Autodesk Inventor part; units mm, degrees
ref_plane "YZ Plane" through (0, 0, 0) normal (1, 0, 0) x (0, 1, 0)
ref_plane "XZ Plane" through (0, 0, 0) normal (0, 1, 0) x (-1, 0, 0)
ref_plane "XY Plane" through (0, 0, 0) normal (0, 0, 1) x (1, 0, 0)
sketch "Sketch1" plane through (0, 0, 0) normal (0, 1, 0) x (-1, 0, 0)
  line L0 (-21.15, 21.15) -> (21.15, 21.15)
  line L1 (21.15, 21.15) -> (21.15, -21.15)
  line L2 (21.15, -21.15) -> (-21.15, -21.15)
  line L3 (-21.15, -21.15) -> (-21.15, 21.15)
  line L4 (-21.15, 21.15) -> (21.15, -21.15) construction
  line L5 (21.15, 21.15) -> (-21.15, -21.15) construction
  line L6 (-15.5, 15.5) -> (15.5, 15.5)
  line L7 (15.5, 15.5) -> (15.5, -15.5)
  line L8 (15.5, -15.5) -> (-15.5, -15.5)
  line L9 (-15.5, -15.5) -> (-15.5, 15.5)
  line L10 (-15.5, 15.5) -> (15.5, -15.5) construction
  line L11 (15.5, 15.5) -> (-15.5, -15.5) construction
  line L12 (15.5, -21.15) -> (21.15, -15.5)
  line L13 (-21.15, -15.5) -> (-15.5, -21.15)
  line L14 (-21.15, 15.5) -> (-15.5, 21.15)
  line L15 (15.5, 21.15) -> (21.15, 15.5)
  point P0 (0, 0)
  dimension "d0" = 42.3
  dimension "d1" = 42.3
  dimension "d2" = 31
  dimension "d3" = 31
  dimension "d4" = 31
  dimension "d5" = 31
  dimension "d6" = 31
  dimension "d7" = 31
  dimension "d8" = 45
extrude "Extrusion1" add sketch "Sketch1" along normal blind 48 contours L0 L15 L1 L12 L2 L13 L3 L14 | L6 L7 L8 L9
sketch "Sketch2" plane through (0, 48, 0) normal (0, 1, 0) x (1, 0, 0)
  circle A0 centre (0, 0) radius 11
  dimension "d11" = 22
extrude "Extrusion2" add sketch "Sketch2" along normal blind 2
sketch "Sketch3" plane through (0, 50, 0) normal (0, 1, 0) x (1, 0, 0)
  circle A0 centre (0, 0) radius 2.5
  dimension "d14" = 5
extrude "Extrusion3" add sketch "Sketch3" along normal blind 22
sketch "Sketch4" plane through (0, 72, 0) normal (0, 1, 0) x (1, 0, 0)
  circle A0 centre (0, 0) radius 2.5
  line L0 (-1.5, 2) -> (1.5, 2)
  circle A1 centre (0, 0) radius 2.5
  dimension "d21" = 5
  dimension "d20" = 2
extrude "Extrusion4" cut sketch "Sketch4" against normal blind 15 contours L0 A0 picked at (-0.3466, 2.0912)
chamfer "Chamfer2" distance 0.2 angle 45 3 edges at (-1.118, 72, 2.2361) (2.2361, 72, -1.118) (0, 72, -2)
sketch "Sketch5" plane through (0, 48, 0) normal (0, 1, 0) x (1, 0, 0)
  circle A0 centre (0, 0) radius 11
  line L0 (-15.5, -21.15) -> (15.5, -21.15)
  line L1 (15.5, -21.15) -> (21.15, -15.5)
  line L2 (21.15, -15.5) -> (21.15, 15.5)
  line L3 (21.15, 15.5) -> (15.5, 21.15)
  line L4 (15.5, 21.15) -> (-15.5, 21.15)
  line L5 (-15.5, 21.15) -> (-21.15, 15.5)
  line L6 (-21.15, 15.5) -> (-21.15, -15.5)
  line L7 (-21.15, -15.5) -> (-15.5, -21.15)
  point P0 (-15.5, 15.5)
  point P1 (15.5, 15.5)
  point P2 (-15.5, -15.5)
  point P3 (15.5, -15.5)
  dimension "d29" = 31
  dimension "d32" = 31
  dimension "d35" = 15.5
  dimension "d36" = 15.5
hole "Hole1" at (-15.5, 48, -15.5) at (15.5, 48, -15.5) at (-15.5, 48, 15.5) at (15.5, 48, 15.5) direction (0, -1, 0) diameter 2.459 depth 4.5 tip angle 118
sketch "Sketch6" plane through (15.5, 0, -21.15) normal (0, 0, -1) x (-1, 0, 0)
  line L0 (0, 0) -> (31, 0)
  line L1 (31, 0) -> (31, 48)
  line L2 (0, 48) -> (31, 48)
  line L3 (0, 0) -> (0, 48)
  line L4 (7.5, 10.5) -> (23.5, 10.5)
  line L5 (23.5, 10.5) -> (23.5, 4.5)
  line L6 (23.5, 4.5) -> (7.5, 4.5)
  line L7 (7.5, 4.5) -> (7.5, 10.5)
  point P0 (15.5, 0)
  dimension "d44" = 16
  dimension "d45" = 6
  dimension "d46" = 10.5
  dimension "d47" = 31
  dimension "d48" = 7.5
extrude "Extrusion5" add sketch "Sketch6" along normal blind 5 contours L4 L5 L6 L7
equation "\"d48\" = -0.5 * d44 + 0.5 * d47"
properties part number "Stepper_NEMA17_48mm"
Design review of the part built by this model. Coordinates are the model's own, in mm. A direction names the side the tool comes from. Round coordinates to 2 decimals unless told otherwise and drop trailing zeros. Write each loop counter-clockwise with the first axis right and the second up, starting at its lowest first coordinate (ties: lowest second). Pieces come first, ordered by that corner, then holes.
Item 1: For probe 1 along Z at (x, y) = (-15.5, 45.15), list the stretches that pass through material, from the lowest coordinate up.
Item 2: We need section B-B on y = 8.5. Write out the cut boundary in (x, z), and give its area (3 significant figures).
Item 3: We need section C-C on z = 0. Write out the cut boundary in (x, y).
Item 4: For faces 1 (the cylindrical face through (-0.33, 60.75, 2.48)), 2 (the flat face through (0, 72, 0)), 3 (the flat face through (0, 10.5, -24)), 4 (the flat face through (0, 4.5, -24)), 5 (the flat face through (18.36, 23.66, 18.29)), list the 3-axis set-ups (+Z, -Z, +X, -X, +Y, -Y) from which the entire face can be reached by the end or side of a thin tool; tool diameter is ignored.
Item 5: Clearance check with flat-ended pins moving along their axes: pin 1 Ø8 at (x, y) = (-2, 59) entering from +Z; pin 2 Ø3 at (x, z) = (-0.5, -16.5) entering from +Y; pin 3 Ø2.5 at (x, z) = (-1, -24) entering from +Y. State where each tip first meets the part, or that it passes through.
Item 6: We need section D-D on y = 39. Write out the cut boundary in (x, z), and give its area (3 significant figures).
Item 7: We need section A-A on x = 0. Write out the cut boundary in (y, z), and give its area (3 significant figures).
Returned:
1. probe 1: z = -21.15 to -16.73, -14.27 to 14.27, 16.73 to 21.15
2. outline: (-21.15, -15.5) - (-15.5, -21.15) - (-8, -21.15) - (-8, -26.15) - (8, -26.15) - (8, -21.15) - (15.5, -21.15) - (21.15, -15.5) - (21.15, 15.5) - (15.5, 21.15) - (-15.5, 21.15) - (-21.15, 15.5) - close
2. area: 1,810 mm2
3. outline: (-21.15, 0) - (21.15, 0) - (21.15, 48) - (11, 48) - (11, 50) - (2.5, 50) - (2.5, 71.8) - (2.3, 72) - (-2.3, 72) - (-2.5, 71.8) - (-2.5, 50) - (-11, 50) - (-11, 48) - (-21.15, 48) - close
4. face 1: +Y
4. face 2: +Z, -Z, +X, -X, +Y
4. face 3: -Z, +X, -X, +Y
4. face 4: -Z, +X, -X, -Y
4. face 5: +Z, +X, +Y, -Y
5. pin 1: stops at z = 2.5
5. pin 2: stops at y = 48
5. pin 3: stops at y = 10.5
6. outline: (-21.15, -15.5) - (-15.5, -21.15) - (15.5, -21.15) - (21.15, -15.5) - (21.15, 15.5) - (15.5, 21.15) - (-15.5, 21.15) - (-21.15, 15.5) - close
6. area: 1,730 mm2
7. outline: (0, -21.15) - (4.5, -21.15) - (4.5, -26.15) - (10.5, -26.15) - (10.5, -21.15) - (48, -21.15) - (48, -11) - (50, -11) - (50, -2.5) - (57, -2.5) - (57, -2) - (71.8, -2) - (72, -1.8) - (72, 2.3) - (71.8, 2.5) - (50, 2.5) - (50, 11) - (48, 11) - (48, 21.15) - (0, 21.15) - close
7. area: 2,210 mm2
